For this review, take the finished solid that the model builds, in its own axes (mm). A direction names the side the tool comes from. Give positions to 0.01 mm unless a question says otherwise; leave off trailing zeros. Loops run counter-clockwise (first coordinate to the right, second up) from the corner with the lowest first, then second, coordinate; pieces in that order, holes last. Notation, with made-up numbers: (6, 54.5) -> (48, 54.5) arc R28 cw to (48, 79.5) -> close; hole circle Ø2 at (63.5, -37). An arc over 180 degrees is marked (long way). One line per question, with ' | ' between items. Start each with the question number.
(1) Wall thickness on probe 1 along X at (y, z) = (-6, 13.5); probe 2 along X at (y, z) = (-4.5, -10.5); probe 3 along Y at (x, z) = (21.5, 9.5): over which ranges is each line inside the solid? List them lowest first.
(2) Insertion check: P1, Ø2.5, axis at x = -28, z = -16.22, coming from the -Y side; P2, Ø15.5, axis at x = -25.5, z = -7.5, coming from the -Y side; P3, Ø1, axis at x = -40.5, y = -11.5, coming from the +Z side; P4, Ø6, axis at x = 5.5, z = -5, coming from the +Y side. Each pin has a flat end and moves straight along its axis. Give the tip position at first contact, or say it passes through.
(3) Consider section C-C (x = -34.5). Write out the cut boundary in (y, z), and give its area (3 significant figures).
(4) Consider section B-B (x = 24). Write out the cut boundary in (y, z).
(5) Consider section A-A (x = -9). Write out the cut boundary in (y, z).
(6) Draft analysis for pull direction X (two halves, no side actions). For faces 5 (the flat face through (-1, -5, -4)), 6 (the flat face through (0, -6, -37.256)), 7 (the flat face through (67.9, -14.3, 32.02)), state which applies: +X half, -X half, draft (parallel to the pull), parting line (faces both ways), or undercut.
(7) Tool access review of faces 1 (the flat face through (-1, -14, 17.191)), 2 (the flat face through (-1, -10, -6)), 3 (the flat face through (39.78, -3.48, 11.35)), 4 (the flat face through (53.657, -8, 10)): name each direction out of +Z, -Z, +X, -X, +Y, -Y from which nothing blocks a thin tool from reaching the whole face with its end or side.
from build123d import *

# Parameters (mm, degrees)
SKETCH_1_R                   = 2
SKETCH_1_R_2                 = 1
EXTRUDE_1_DEPTH              = 29
CUT_EXTRUDE_1_DEPTH          = 5
CUT_EXTRUDE_START            = -10
CUT_EXTRUDE_2_DEPTH          = 19
CUT_EXTRUDE_3_DEPTH          = 2
SKETCH_11_R                  = 1.5
CUT_EXTRUDE_4_DEPTH          = 104.437531222
SKETCH_13_R                  = 1.25
CUT_EXTRUDE_5_DEPTH          = 2
HOLE_WIZARD_M2_5_6_D         = 2.05
HOLE_WIZARD_M3_1_D           = 2.5
HOLE_WIZARD_M3_1_CSINK_D     = 3.05
HOLE_WIZARD_M3_1_CSINK_ANGLE = 90
CHAMFER_1_SIZE               = 2
FILLET_1_R                   = 3
FILLET_2_R                   = 1


with BuildPart() as part:
    # 草图1 → 凸台-拉伸1 (new body)
    # profile 1 of 2: a face of its own
    with BuildSketch(Plane(origin=(0, 0, 0), x_dir=(1, 0, 0), z_dir=(0, 1, 0))):
        Polygon((69.296464556, -30.626082539), (66.468037432, -33.454509664), (50.204581464, -17.191053697), (47.376154339, -20.019480821), (43.376154339, -20.019480821), (40.547727215, -17.191053697), (2.052219297, -17.191053697), (-40.547727215, -17.191053697), (-43.376154339, -20.019480821), (-47.376154339, -20.019480821), (-50.204581464, -17.191053697), (-66.468037432, -33.454509664), (-69.296464556, -30.626082539), (-53.656854249, -14.986472232), (-53.656854249, -3.776840134), (-28, 21.880014115), (-16.790367902, 21.880014115), (0, 38.670382017), (16.790367902, 21.880014115), (28, 21.880014115), (53.656854249, -3.776840134), (53.656854249, -14.986472232), align=None)
        with Locations(Location((28, 16.223159866, 0), (0, 0, 270))):
            Circle(SKETCH_1_R, mode=Mode.SUBTRACT)
        with Locations(Location((-28, 16.223159866, 0), (0, 0, 270))):
            Circle(SKETCH_1_R, mode=Mode.SUBTRACT)
        with Locations(Location((-48, -3.776840134, 0), (0, 0, 270))):
            Circle(SKETCH_1_R, mode=Mode.SUBTRACT)
        with Locations((44.194173824, -11.180646057)):
            Circle(SKETCH_1_R_2, mode=Mode.SUBTRACT)
        with Locations((-44.194173824, -11.180646057)):
            Circle(SKETCH_1_R_2, mode=Mode.SUBTRACT)
        with Locations((0, 33.013527768)):
            Circle(SKETCH_1_R_2, mode=Mode.SUBTRACT)
        with Locations(Location((48, -3.776840134, 0), (0, 0, 270))):
            Circle(SKETCH_1_R, mode=Mode.SUBTRACT)
        Polygon((-43.487067043, -7.645112151), (-37.355339059, -13.776840134), (37.355339059, -13.776840134), (43.487067043, -7.645112151), (5.828427125, 30.013527768), (-5.828427125, 30.013527768), align=None, mode=Mode.SUBTRACT)
    # profile 2 of 2: a face of its own
    with BuildSketch(Plane(origin=(0, 0, 0), x_dir=(1, 0, 0), z_dir=(0, 1, 0))):
        Polygon((-5.828427125, 30.013527768), (-43.487067043, -7.645112151), (-37.355339059, -13.776840134), (37.355339059, -13.776840134), (43.487067043, -7.645112151), (5.828427125, 30.013527768), align=None)
    extrude(amount=-EXTRUDE_1_DEPTH)

    # 草图1<3> → 切除-拉伸1 (cut)
    with BuildSketch(Plane(origin=(0, 0, 0), x_dir=(1, 0, 0), z_dir=(0, 1, 0))):
        Polygon((-5.828427125, 30.013527768), (-43.487067043, -7.645112151), (-37.355339059, -13.776840134), (37.355339059, -13.776840134), (43.487067043, -7.645112151), (5.828427125, 30.013527768), align=None)
    extrude(amount=-CUT_EXTRUDE_1_DEPTH, mode=Mode.SUBTRACT)

    # 草图3 → 切除-拉伸2 (cut)
    with BuildSketch(Plane(origin=(0, 0, 0), x_dir=(1, 0, 0), z_dir=(0, 1, 0)).offset(CUT_EXTRUDE_START)):
        Polygon((-74.127206293, -13.776840134), (70.632375227, -13.776840134), (4.598461929, 56.317971506), align=None)
    extrude(amount=-CUT_EXTRUDE_2_DEPTH, mode=Mode.SUBTRACT)

    # 草图4 → 切除-拉伸3 (cut)
    with BuildSketch(Plane(origin=(0, 0, 0), x_dir=(1, 0, 0), z_dir=(0, 1, 0))):
        with BuildLine():
            Line((-2.121320344, 36.549061673), (-48.535533906, -9.865151889))
            ThreePointArc((-48.535533906, -9.865151889), (-49.18585216, -13.13452253), (-46.414213562, -14.986472232))
            Line((-46.414213562, -14.986472232), (46.414213562, -14.986472232))
            ThreePointArc((46.414213562, -14.986472232), (49.18585216, -13.13452253), (48.535533906, -9.865151889))
            Line((48.535533906, -9.865151889), (0, 38.670382017))
            Line((0, 38.670382017), (-2.121320344, 36.549061673))
        make_face()
    extrude(amount=-CUT_EXTRUDE_3_DEPTH, mode=Mode.SUBTRACT)

    # 草图11 → 切除-拉伸4 (cut, through all)
    with BuildSketch(Plane(origin=(-16.506763884, 0, -16.506763884), x_dir=(0.7071067811865477, 0, -0.7071067811865474), z_dir=(0.7071067811865474, 0, 0.7071067811865477))):
        with Locations((-52.155910645, -9.5)):
            Circle(SKETCH_11_R)
        with Locations((-52.155910645, -19.5)):
            Circle(SKETCH_11_R)
        with Locations((-67.155910645, -19.5)):
            Circle(SKETCH_11_R)
        with Locations((-67.155910645, -9.5)):
            Circle(SKETCH_11_R)
    cut_extrude_4 = extrude(amount=-CUT_EXTRUDE_4_DEPTH, mode=Mode.SUBTRACT)

    # 草图13 → 切除-拉伸5 (cut)
    with BuildSketch(Plane(origin=(-19.335191009, 0, -19.335191009), x_dir=(-0.7071067811865488, 0, 0.7071067811865462), z_dir=(-0.7071067811865462, 0, -0.7071067811865488))):
        with Locations((59.597036142, -26)):
            Circle(SKETCH_13_R)
    cut_extrude_5 = extrude(amount=-CUT_EXTRUDE_5_DEPTH, mode=Mode.SUBTRACT)

    # M2.5 螺纹孔6 (through all)
    with Locations(Plane(origin=(0, -2, -33.013527768), x_dir=(0, 0, 1), z_dir=(0, 1, 0))):
        with Locations((0, 0), (44.194173825, -44.194173824), (44.194173825, 44.194173824)):
            Hole(HOLE_WIZARD_M2_5_6_D / 2)

    # M3 螺纹孔1 (through all)
    with Locations(Plane(origin=(-61.476659403, -26, 22.806277386), x_dir=(-0.707106781187, 0, 0.707106781187), z_dir=(-0.707106781187, 0, -0.707106781187))):
        with Locations((0, 0)):
            hole_wizard_m3_1 = CounterSinkHole(HOLE_WIZARD_M3_1_D / 2, HOLE_WIZARD_M3_1_CSINK_D / 2, counter_sink_angle=HOLE_WIZARD_M3_1_CSINK_ANGLE)

    # 镜向2: 切除-拉伸4, 切除-拉伸5, M3 螺纹孔1 across plane
    add(cut_extrude_4.mirror(Plane.ZY), mode=Mode.SUBTRACT)
    add(cut_extrude_5.mirror(Plane.ZY), mode=Mode.SUBTRACT)
    add(hole_wizard_m3_1.mirror(Plane.ZY), mode=Mode.SUBTRACT)

    # 倒角1
    chamfer_1_edges = [part.edges().sort_by_distance(p)[0] for p in [
        (0, -6, -38.670382017),
    ]]
    chamfer(chamfer_1_edges, length=CHAMFER_1_SIZE)

    # 圆角1
    fillet_1_edges = [part.edges().sort_by_distance(p)[0] for p in [
        (-16.790367902, -6, -21.880014115),
        (16.790367902, -6, -21.880014115),
        (-43.487067043, -3.5, 7.645112151),
        (-5.828427125, -3.5, -30.013527768),
        (-37.355339059, -3.5, 13.776840134),
        (5.828427125, -3.5, -30.013527768),
        (37.355339059, -3.5, 13.776840134),
        (43.487067043, -3.5, 7.645112151),
        (-40.547727215, -14.5, 17.191053697),
        (40.547727215, -14.5, 17.191053697),
    ]]
    fillet(fillet_1_edges, radius=FILLET_1_R)

    # 圆角2
    fillet_2_edges = [part.edges().sort_by_distance(p)[0] for p in [
        (-53.656854249, -14.5, 14.986472232),
        (53.656854249, -14.5, 14.986472232),
        (-50.204581464, -14.5, 17.191053697),
        (50.204581464, -14.5, 17.191053697),
    ]]
    fillet(fillet_2_edges, radius=FILLET_2_R)


solid = part.part
A:
1) probe 1: x = -53.66 to 53.66 | probe 2: x = -39.38 to -25.34, 25.34 to 39.38 | probe 3: y = -10 to -5
2) P1: passes through | P2: stops at y = -10 | P3: stops at z = 17.72 | P4: stops at y = -5
3) outline: (-29, 13.78) -> (-10, 13.78) -> (-10, -15.38) -> (0, -15.38) -> (0, -4.17) -> (-2, -4.17) -> (-2, -1.34) -> (-5, -1.34) -> (-5, 13.78) -> (-2, 13.78) -> (-2, 14.99) -> (0, 14.99) -> (0, 17.19) -> (-29, 17.19) -> close | area: 307 mm^2
4) outline: (-29, 13.78) -> (-10, 13.78) -> (-10, -21.88) -> (0, -21.88) -> (0, -14.67) -> (-2, -14.67) -> (-2, -11.84) -> (-5, -11.84) -> (-5, 13.78) -> (-2, 13.78) -> (-2, 14.99) -> (0, 14.99) -> (0, 17.19) -> (-29, 17.19) -> close
5) outline: (-29, 13.78) -> (-10, 13.78) -> (-10, -29.67) -> (-2, -29.67) -> (-2, -26.84) -> (-5, -26.84) -> (-5, 13.78) -> (-2, 13.78) -> (-2, 14.99) -> (0, 14.99) -> (0, 17.19) -> (-29, 17.19) -> close
6) face 5: undercut | face 6: draft | face 7: +X half
7) face 1: +Z, +Y, -Y | face 2: -Z, +X, -X, -Y | face 3: +Y | face 4: -Z, +X, +Y, -Y
